Could you check a few things on this model? Use its own coordinates, in mm. Face numbers are marked on the shaded views. A direction names the side the tool comes from. Coordinates: 2 decimals unless noted, no trailing zeros. Order: outer loops, then holes, each group sorted by start corner. A loop starts at its lowest first (then second) coordinate and runs counter-clockwise, first axis right, second up. Notation, with made-up numbers: (53.25, -8.5) -> (110.25, -8.5) arc R19 cw to (110.25, 28.5) -> close; hole circle Ø9 at (-27, -12). An arc over 180 degrees is marked (long way). Put each result on its own line as item: value. Start each with the question number.
Q1. We'd pull the mould along Z, two halves only. Please class the marked faces 4, 5 and 6: +Z half, -Z half, draft (parallel to the pull), parting line (faces both ways), or undercut.
Q2. Will these pins go through, and if not, where does the flat tip stop? pin 1 (3 mm diameter, centred on x = 3, z = 1, fed in from +Y); pin 2 (6 mm diameter, centred on x = -4, z = -6, fed in from -Y); pin 3 (5 mm diameter, centred on x = 4, z = 0, fed in from -Y).
Q3. For the marked faces 1, 2 and 3, which set-ups out of +Z, -Z, +X, -X, +Y, -Y let a thin tool reach every point of the face, with its end or its side?
Q4. If we section it at B-B (z = -2.5): Please give me the cut outline in (x, y), and give its area (3 significant figures).
Q5. If we section it at C-C (y = 2): Please give me the cut outline in (x, z).
Q6. Please list where these lines run through material, in increasing order: line 1 along Y through (x, z) = (0, 9.45); line 2 along X through (y, z) = (0.5, 3).
Q7. If we section it at A-A (y = 0): Please give me the cut outline in (x, z).
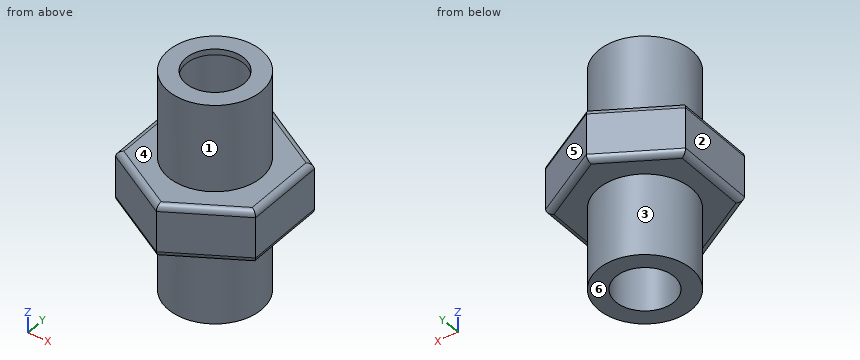
Autodesk Inventor part; units mm, degrees
ref_plane "YZ Plane" through (0, 0, 0) normal (1, 0, 0) x (0, 1, 0)
ref_plane "XZ Plane" through (0, 0, 0) normal (0, 1, 0) x (-1, 0, 0)
ref_plane "XY Plane" through (0, 0, 0) normal (0, 0, 1) x (1, 0, 0)
sketch "Sketch1" plane through (0, 0, 0) normal (0, 0, 1) x (1, 0, 0)
  line L0 (0, -6.9282) -> (-6, -3.4641)
  line L1 (-6, -3.4641) -> (-6, 3.4641)
  line L2 (-6, 3.4641) -> (0, 6.9282)
  line L3 (0, 6.9282) -> (6, 3.4641)
  line L4 (6, 3.4641) -> (6, -3.4641)
  line L5 (6, -3.4641) -> (0, -6.9282)
  circle A0 centre (0, 0) radius 4
  dimension "d0" = 12
  dimension "d1" = 8
extrude "Extrusion1" add sketch "Sketch1" along normal mid plane 4.5 contours L0 L1 L2 L3 L4 L5 | A0
extrude "Extrusion2" add sketch "Sketch1" along normal mid plane 18.5 contours A0
thread "Thread1"
sketch "Sketch2" plane through (0, 0, -9.25) normal (0, 0, -1) x (-1, 0, 0)
  point P0 (0, 0)
hole "Hole1" at (0, 0, -9.25) direction (0, 0, 1) diameter 5 end through all
fillet "Fillet1" radius 0.5 12 edges at (-6, 0, -2.25) (-3, -5.1962, -2.25) (3, -5.1962, -2.25) (-3, 5.1962, -2.25) (6, 0, -2.25) (3, 5.1962, -2.25) (-3, 5.1962, 2.25) (3, 5.1962, 2.25) (6, 0, 2.25) (3, -5.1962, 2.25) (-3, -5.1962, 2.25) (-6, 0, 2.25)
sketch "Sketch3" plane through (0, 0, 9.25) normal (0, 0, 1) x (1, 0, 0)
  circle A0 centre (0, 0) radius 4
  circle A1 centre (0, 0) radius 2.5
  dimension "d16" = 8
  dimension "d17" = 5
extrude "Extrusion3" add sketch "Sketch3" along normal blind 0.5
thread "Thread2"
properties part number "HUDSON-1-82"
The answers:
1. face 4: +Z half
1. face 5: draft
1. face 6: -Z half
2. pin 1: y = 6.06
2. pin 2: y = -3.87
2. pin 3: y = -6.06
3. face 1: +Z
3. face 2: +Z, -Z, -X, +Y, -Y
3. face 3: -Z
4. outline: circle Ø8 at (0, 0); hole circle Ø5 at (0, 0)
4. area: 30.6 mm^2
5. outline: (-6, -1.75) arc R0.5 ccw to (-5.5, -2.25) -> (-3.46, -2.25) -> (-3.46, -9.25) -> (-1.5, -9.25) -> (-1.5, 9.75) -> (-3.46, 9.75) -> (-3.46, 2.25) -> (-5.5, 2.25) arc R0.5 ccw to (-6, 1.75) -> close; (1.5, -9.25) -> (3.46, -9.25) -> (3.46, -2.25) -> (5.5, -2.25) arc R0.5 ccw to (6, -1.75) -> (6, 1.75) arc R0.5 ccw to (5.5, 2.25) -> (3.46, 2.25) -> (3.46, 9.75) -> (1.5, 9.75) -> close
6. line 1: -4 to -2.5, 2.5 to 4
6. line 2: -3.97 to -2.45, 2.45 to 3.97
7. outline: (-6, -1.75) arc R0.5 ccw to (-5.5, -2.25) -> (-4, -2.25) -> (-4, -9.25) -> (-2.5, -9.25) -> (-2.5, 9.75) -> (-4, 9.75) -> (-4, 2.25) -> (-5.5, 2.25) arc R0.5 ccw to (-6, 1.75) -> close; (2.5, -9.25) -> (4, -9.25) -> (4, -2.25) -> (5.5, -2.25) arc R0.5 ccw to (6, -1.75) -> (6, 1.75) arc R0.5 ccw to (5.5, 2.25) -> (4, 2.25) -> (4, 9.75) -> (2.5, 9.75) -> close
